from build123d import *

# Parameters (mm, degrees)
F1_DEPTH = 50.8
F2_W     = 12.7
F2_H     = 152.4
F3_DEPTH = 6.35


# Not quite as in the source:
# - a feature names something its author has since deleted; it is built from what else it names


with BuildPart() as f1:
    # F0 (on Front) → F1 (new body)
    with BuildSketch(Plane.XZ):
        Polygon((50.8, 0), (0, 0), (0, -1016), (25.4, -1016), (50.8, -381), align=None)
    extrude(amount=-F1_DEPTH)

    # F2 (on face) → F3 (cut)
    with BuildSketch(Plane.YZ.offset(50.8)):
        with Locations((19.05, -76.2)):
            Rectangle(F2_W, F2_H)
    extrude(amount=-F3_DEPTH, mode=Mode.SUBTRACT)


solid = f1.part
Here's how the part is built. I have some questions about the finished solid (model axes, mm). Round coordinates to 2 decimals unless told otherwise and drop trailing zeros. Loops run counter-clockwise (first coordinate to the right, second up) from the corner with the lowest first, then second, coordinate; pieces in that order, holes last. Notation, with made-up numbers: (-23, 43.5) - (6, 43.5) arc R19 ccw to (6, 75.5) - close; hole circle Ø4 at (76.25, 43.5). An arc over 180 degrees is marked (long way). One line per question, with ' | ' between items. Start each with the question number.
Q1. Will this pin go through, and if not, where does the flat tip stop? pin 1 (4 mm diameter, centred on y = 22, z = -59, fed in from +X).
Q2. I want a section at C-C (x = 35.5). Write out the boundary of the cut face in (y, z), then the cut area to 3 significant figures.
Q3. Please list where these lines run through material, in increasing order: line 1 (X direction, y = 35, z = -624.5); line 2 (X direction, y = 39.5, z = -431.5). Write a range as [from, to].
Q4. I want a section at A-A (y = 34). Write out the boundary of the cut face in (x, z), then the cut area to 3 significant figures.
Q5. I want a section at B-B (z = -715). Write out the boundary of the cut face in (x, y), then the cut area to 3 significant figures.
Response values:
1) pin 1: stops at x = 44.45
2) outline: (0, -763.5) - (50.8, -763.5) - (50.8, 0) - (0, 0) - close | area: 38,800 mm²
3) line 1: x = [0, 41.06] | line 2: x = [0, 48.78]
4) outline: (0, -1016) - (25.4, -1016) - (50.8, -381) - (50.8, 0) - (0, 0) - close | area: 43,500 mm²
5) outline: (0, 0) - (37.44, 0) - (37.44, 50.8) - (0, 50.8) - close | area: 1,900 mm²
